Read the model definition and answer for the solid it produces. Units are mm, in the model's axes. A direction names the side the tool comes from. Coordinates: 2 decimals unless noted, no trailing zeros. Order: outer loops, then holes, each group sorted by start corner. A loop starts at its lowest first (then second) coordinate and runs counter-clockwise, first axis right, second up. Notation, with made-up numbers: M 74,27.25 L 93,27.25 A29 ccw 93,47.25 Z; hole C -28.75,74 d4. An arc over 180 degrees is marked long. Use a Markdown table: item, result. Add a question column.
1) Each of these flat-tipped pins is pushed along its axis until it touches: pin 1 Ø4 at (x, z) = (-2.5, 77) entering from -Y; pin 2 Ø1.5 at (x, z) = (2, 93.5) entering from -Y; pin 3 Ø2 at (y, z) = (0.5, 58.5) entering from +X. Where does it stop, or does it pass through?
2) Find the intervals of material crossed by probe 1 along Y at (x, z) = (-1.5, 109.5); probe 2 along X at (y, z) = (0.25, 41.5); probe 3 along Y at (x, z) = (0.5, 107), in increasing order. Write a range as [from, to].
3) Find section C-C on z = 67. Write down the section's boundary in (x, y), plus the area to 3 significant figures.
4) For faces 4 (the face through (3.8, -3.5, 0)), 5 (the face through (-3.47, -3.6, 9.86)), 6 (the face through (-3.8, 3.5, 0)), 7 (the face through (0, 5, -2)), 8 (the face through (-2, 4, 71)), determine the directions among +Z, -Z, +X, -X, +Y, -Y from which every point of the face is accessible in a straight line to the end or side of a thin tool.
5) Find section B-B on x = 0. Write down the section's boundary in (y, z), plus the area to 3 significant figures.
6) Find section A-A on y = 0. Write down the section's boundary in (x, z).
7) The mould has two halves that part along X. Classify faces 1 (the face through (0, 4, 20)), 2 (the face through (4.9, 1.6, 20)), 3 (the face through (0, -5, 71)): released by +X, released by -X, zero draft, split by the parting line, or undercut.
from build123d import *

# Parameters (mm, degrees)
EXTRUDE_1_DEPTH     = 20
SKETCH_2_R          = 5
EXTRUDE_2_DEPTH     = 5
EXTRUDE_START       = 100
SKETCH_7_R          = 5
EXTRUDE_4_DEPTH     = 100
SKETCH_8_W          = 4
SKETCH_8_H          = 3
CUT_EXTRUDE_1_DEPTH = 100


with BuildPart() as part:
    # 草图1 → 凸台-拉伸1 (new body)
    with BuildSketch(Plane.XY):
        Polygon((5.536193055, 1.63826121), (1.349320701, 5.613614431), (-4.186872353, 3.975353221), (-5.536193055, -1.63826121), (-1.349320701, -5.613614431), (4.186872353, -3.975353221), align=None)
    extrude(amount=EXTRUDE_1_DEPTH)

    # 草图2 → 凸台-拉伸2 (add)
    with BuildSketch(Plane(origin=(0, 0, 0), x_dir=(-1, 0, 0), z_dir=(0, 0, -1))):
        with Locations(Location((0, 0, 0), (0, 0, 193.51554681))):
            Circle(SKETCH_2_R)
    extrude(amount=EXTRUDE_2_DEPTH)

    # 草图7 → 凸台-拉伸4 (add)
    with BuildSketch(Plane.XY.offset(20).offset(EXTRUDE_START)):
        with Locations(Location((0, 0, 0), (0, 0, 346.48445319))):
            Circle(SKETCH_7_R)
    extrude(amount=-EXTRUDE_4_DEPTH)

    # 草图8 → 切除-拉伸1 (cut)
    with BuildSketch(Plane.XY.offset(120)):
        with Locations((0, 4.082575695)):
            Rectangle(SKETCH_8_W, SKETCH_8_H)
    extrude(amount=-CUT_EXTRUDE_1_DEPTH, mode=Mode.SUBTRACT)


solid = part.part
Check result:
| question | item | result |
|---|---|---|
| 1 | pin 1 | stops at y = -4.97 |
| 1 | pin 2 | stops at y = -4.84 |
| 1 | pin 3 | stops at x = 5 |
| 2 | probe 1 | y = [-4.77, 2.58] |
| 2 | probe 2 | x = [-4.99, 4.99] |
| 2 | probe 3 | y = [-4.97, 2.58] |
| 3 | outline | M -2,2.58 L -2,4.58 A5 ccw long 2,4.58 L 2,2.58 Z |
| 3 | area | 69.4 mm2 |
| 4 | face 4 | -Z, +X, -Y |
| 4 | face 5 | +Z, -Z, -X, -Y |
| 4 | face 6 | -Z, -X, +Y |
| 4 | face 7 | -Z |
| 4 | face 8 | +Z, +Y |
| 5 | outline | M -5.21,0 L -5,0 L -5,-5 L 5,-5 L 5,0 L 5.21,0 L 5.21,20 L 2.58,20 L 2.58,120 L -5,120 L -5,20 L -5.21,20 Z |
| 5 | area | 1,020 mm2 |
| 6 | outline | M -5.14,0 L -5,0 L -5,-5 L 5,-5 L 5,0 L 5.14,0 L 5.14,20 L 5,20 L 5,120 L -5,120 L -5,20 L -5.14,20 Z |
| 7 | face 1 | undercut |
| 7 | face 2 | zero draft |
| 7 | face 3 | split by the parting line |
